Drawing for the job (mm, zero at the part's lowest x, y, z). A direction names the side the tool comes from. Give positions to 0.01 mm unless a question says otherwise; leave off trailing zeros. Order: outer loops, then holes, each group sorted by start corner. A loop starts at its lowest first (then second) coordinate and runs counter-clockwise, first axis right, second up. Notation, with made-up numbers: (16, -7.75) - (22, -7.75) arc R23 cw to (22, 17.25) - close; hole circle Ø8 at (-14, -21.75). An arc over 180 degrees is marked (long way). Use a Markdown table: item, result. Add a question column.
(1) Flat gauge pins, fed straight in: pin 1 (2.5 mm diameter, centred on x = 48.5, y = 4, fed in from +Z); pin 2 (4 mm diameter, centred on x = 45, z = 4, fed in from -Y); pin 3 (0.6 mm diameter, centred on x = 71.5, y = 10, fed in from +Z). Where does each tip first touch, or does it go through?
(2) Slice it at D-D (x = 69). Write the cut outline in (y, z), then the cut area to 3 significant figures.
(3) Wall check: line 1 (Z direction, x = 8, y = 5.5); line 2 (Y direction, x = 18, z = 5.5). Give the ranges that are in metal, low to high.
(4) Slice it at C-C (z = 5.5). Write the cut outline in (x, y), then the cut area to 3 significant figures.
(5) Which spindle directions (+Z, -Z, +X, -X, +Y, -Y) get a long thin tool onto all of the face, cutting with end or side? Do the marked faces 1, 2 and 3. Say none if no direction does.
(6) Slice it at B-B (y = 15.25). Write the cut outline in (x, z).
(7) Slice it at A-A (x = 10). Write the cut outline in (y, z).
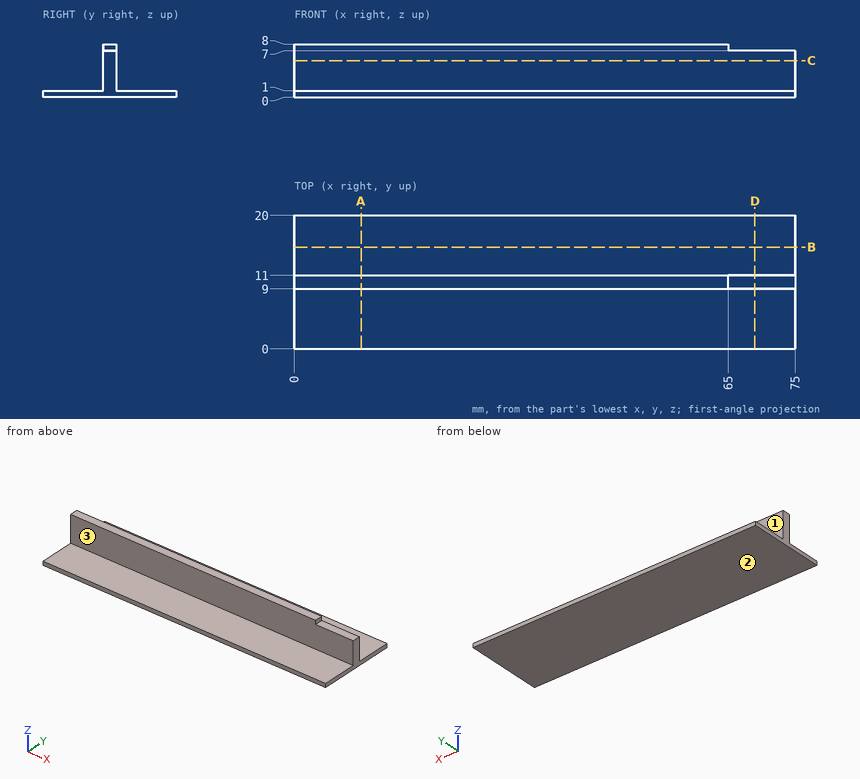
Solution:
| question | item | result |
|---|---|---|
| 1 | pin 1 | z = 1 |
| 1 | pin 2 | y = 9 |
| 1 | pin 3 | z = 7 |
| 2 | outline | (0, 0) - (20, 0) - (20, 1) - (11, 1) - (11, 7) - (9, 7) - (9, 1) - (0, 1) - close |
| 2 | area | 32.0 mm2 |
| 3 | line 1 | 0 to 1 |
| 3 | line 2 | 9 to 11 |
| 4 | outline | (0, 9) - (75, 9) - (75, 11) - (0, 11) - close |
| 4 | area | 150 mm2 |
| 5 | face 1 | +Z, +X, -X, +Y |
| 5 | face 2 | -Z, +X, -X, +Y, -Y |
| 5 | face 3 | +Z, +X, -X, -Y |
| 6 | outline | (0, 0) - (75, 0) - (75, 1) - (0, 1) - close |
| 7 | outline | (0, 0) - (20, 0) - (20, 1) - (11, 1) - (11, 8) - (9, 8) - (9, 1) - (0, 1) - close |
